Here's how the part is built. I have some questions about the finished solid (model axes, mm). A direction names the side the tool comes from. Coordinates: 2 decimals unless noted, no trailing zeros. Loops run counter-clockwise (first coordinate to the right, second up) from the corner with the lowest first, then second, coordinate; pieces in that order, holes last.
```python
from build123d import *

# Parameters (mm, degrees)
PAD_DEPTH       = 40
SKETCH001_W     = 14.5
SKETCH001_H     = 37
POCKET_DEPTH    = 64
SKETCH002_R     = 2
POCKET001_DEPTH = 5
FILLET_R        = 1
FILLET001_R     = 1
CHAMFER_SIZE    = 0.5
CHAMFER001_SIZE = 2


with BuildPart() as part:
    # Sketch → Pad (new body)
    with BuildSketch(Plane.XZ):
        Polygon((0, 0), (0, 19.5), (66.5, 19.5), (66.5, 3), (100, 3), (100, 0), align=None)
    extrude(amount=PAD_DEPTH)

    # Sketch001 (on Face3 of Pad) → Pocket (cut)
    with BuildSketch(Plane(origin=(66.5, 0, 0), x_dir=(0, 0, 1), z_dir=(1, 0, 0))):
        with Locations((10.25, 19.980706)):
            Rectangle(SKETCH001_W, SKETCH001_H)
    extrude(amount=-POCKET_DEPTH, mode=Mode.SUBTRACT)

    # Sketch002 (on Face12 of Pocket) → Pocket001 (cut)
    with BuildSketch(Plane(origin=(0, 0, 3), x_dir=(-1, 0, 0), z_dir=(0, 0, 1))):
        with Locations((-90, 30)):
            Circle(SKETCH002_R)
        with Locations((-90, 10)):
            Circle(SKETCH002_R)
    extrude(amount=-POCKET001_DEPTH, mode=Mode.SUBTRACT)

    # Fillet
    fillet_edges = [part.edges().sort_by_distance(p)[0] for p in [
        (33.25, 0, 19.5),
        (33.25, -40, 19.5),
    ]]
    fillet(fillet_edges, radius=FILLET_R)

    # Fillet001
    fillet001_edges = [part.edges().sort_by_distance(p)[0] for p in [
        (100, 0, 1.5),
        (100, -40, 1.5),
    ]]
    fillet(fillet001_edges, radius=FILLET001_R)

    # Chamfer
    chamfer_edges = [part.edges().sort_by_distance(p)[0] for p in [
        (66.5, -38.480706, 10.25),
        (66.5, -19.980706, 17.5),
        (66.5, -1.480706, 10.25),
    ]]
    chamfer(chamfer_edges, length=CHAMFER_SIZE)

    # Chamfer001
    chamfer001_edges = [part.edges().sort_by_distance(p)[0] for p in [
        (92, -10, 3),
        (92, -30, 3),
    ]]
    chamfer(chamfer001_edges, length=CHAMFER001_SIZE)


solid = part.part
```
1. I want a section at A-A (x = 90). Please give me the cut outline in (y, z).
2. We'd pull the mould along Y, two halves only. Please class faces 4 (the flat face through (2.5, -20, 10)), 5 (the flat face through (39, 0, 9)), 6 (the flat face through (33, -20, 19.5)): +Y half, -Y half, draft (parallel to the pull), parting line (faces both ways), or undercut.
3. For pin 1 (2 mm diameter, centred on y = -7, z = 14.5, fed in from +X), with a flat end and sliding along its axis, tell me the tip position at first contact or that it passes through.
4. I want a section at B-B (y = -30). Please give me the cut outline in (x, z), then the cut area to 3 significant figures.
5. I want a section at D-D (z = 7.5). Please give me the cut outline in (x, y).
6. I want a section at C-C (x = 44.5). Please give me the cut outline in (y, z), then the cut area to 3 significant figures.
7. On a 3-axis mill with a long thin cutter (end or side, diameter ignored), from which of +Z, -Z, +X, -X, +Y, -Y can I reach the whole of each face in a straight line? I mean faces 1 (the flat face through (35, -20, 17.5)), 2 (the cylindrical face through (88.153, -29.234, 0.507)), 3 (the flat face through (66.5, -20, 19)). Say none if no direction works.
8. I need wall thicknesses on line 1 along Y through (x, z) = (90, 0.35); line 2 along Z through (x, y) = (17, -29); line 3 along X through (y, z) = (-10, 0.35). Which ranges of each line are inside material? Lowest first, please.
Response values:
1. outline: (-40, 0) - (-32, 0) - (-32, 1) - (-34, 3) - (-40, 3) - close; (-28, 0) - (-12, 0) - (-12, 1) - (-14, 3) - (-26, 3) - (-28, 1) - close; (-8, 0) - (0, 0) - (0, 3) - (-6, 3) - (-8, 1) - close
2. face 4: undercut
2. face 5: +Y half
2. face 6: draft
3. pin 1: stops at x = 2.5
4. outline: (0, 0) - (88, 0) - (88, 1) - (86, 3) - (2.5, 3) - (2.5, 17.5) - (66, 17.5) - (66.5, 18) - (66.5, 19.5) - (0, 19.5) - close; (92, 0) - (100, 0) - (100, 3) - (94, 3) - (92, 1) - close
4. area: 453 mm2
5. outline: (0, -40) - (66.5, -40) - (66.5, -38.98) - (66, -38.48) - (2.5, -38.48) - (2.5, -1.48) - (66, -1.48) - (66.5, -0.98) - (66.5, 0) - (0, 0) - close
6. outline: (-40, 0) - (0, 0) - (0, 18.5) arc R1 ccw to (-1, 19.5) - (-39, 19.5) arc R1 ccw to (-40, 18.5) - close; hole (-38.48, 3) - (-1.48, 3) - (-1.48, 17.5) - (-38.48, 17.5) - close
6. area: 243 mm2
7. face 1: +X
7. face 2: +Z, -Z
7. face 3: +Z, +X, +Y, -Y
8. line 1: y = -40 to -32, -28 to -12, -8 to 0
8. line 2: z = 0 to 3, 17.5 to 19.5
8. line 3: x = 0 to 88, 92 to 100
